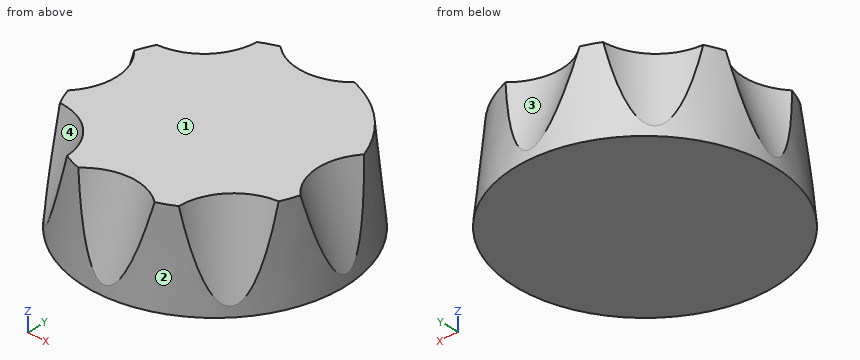
from build123d import *

# Parameters (mm, degrees)
REVOLVE1_ANGLE     = 19.5
CUT_EXTRUDE3_DEPTH = 30
REVOLVE2_ANGLE     = 19.5
CUT_EXTRUDE4_DEPTH = 30
REVOLVE3_ANGLE     = 19.5
CUT_EXTRUDE5_DEPTH = 30
REVOLVE4_ANGLE     = 19.5
CUT_EXTRUDE6_DEPTH = 30
REVOLVE5_ANGLE     = 19.5
CUT_EXTRUDE7_DEPTH = 30
REVOLVE6_ANGLE     = 19.5
CUT_EXTRUDE8_DEPTH = 30
REVOLVE7_ANGLE     = 19.5
CUT_EXTRUDE9_DEPTH = 30


# Read off the part's stored shape, not the designer's step: Boundary1
with BuildPart() as part:
    # Boundary1 outline → Boundary1 (revolve)
    with BuildSketch(Plane.XZ):
        Polygon((23.4, 0), (21.75, 16.55), (0, 16.55), (0, 0), align=None)
    revolve(axis=Axis((0, 0, 0), (0, 0, 1)))

    # Sketch3 → Revolve1 (revolve)
    with BuildSketch(Plane.XY.offset(16.55)):
        with BuildLine():
            ThreePointArc((6.7, 20.692329497), (0, 21.75), (-6.7, 20.692329497))
            ThreePointArc((-6.7, 20.692329497), (0, 18.897069907), (6.7, 20.692329497))
        make_face()
    revolve(axis=Axis((-21.75, 0, 16.55), (1, 0, 0)), revolution_arc=REVOLVE1_ANGLE)

    # Sketch21 → Cut-Extrude3 (cut)
    # profile 1 of 2: a face of its own
    with BuildSketch(Plane(origin=(0, -5.207626236, 14.705882831), x_dir=(1, 0, 0), z_dir=(0, -0.3338068592337716, 0.9426414910921781))):
        with BuildLine():
            Line((9.372530559, 28.241040631), (-9.372530559, 28.241040631))
            ThreePointArc((-9.372530559, 28.241040631), (0, 22.47450352), (9.372530559, 28.241040631))
        make_face()
        with BuildLine():
            ThreePointArc((6.7, 26.216833017), (0, 24.421573428), (-6.7, 26.216833017))
            ThreePointArc((-6.7, 26.216833017), (0, 27.27450352), (6.7, 26.216833017))
        make_face(mode=Mode.SUBTRACT)
    # profile 2 of 2: a face of its own
    with BuildSketch(Plane(origin=(0, -5.207626236, 14.705882831), x_dir=(1, 0, 0), z_dir=(0, -0.3338068592337716, 0.9426414910921781))):
        with BuildLine():
            ThreePointArc((6.7, 26.216833017), (0, 27.27450352), (-6.7, 26.216833017))
            ThreePointArc((-6.7, 26.216833017), (0, 24.421573428), (6.7, 26.216833017))
        make_face()
    extrude(amount=-CUT_EXTRUDE3_DEPTH, mode=Mode.SUBTRACT)

    # Sketch22 → Revolve2 (revolve)
    with BuildSketch(Plane.XY.offset(16.55)):
        with BuildLine():
            ThreePointArc((-19.454905378, 9.724667435), (-15.513197269, 15.244776499), (-10.062721237, 19.282223454))
            ThreePointArc((-10.062721237, 19.282223454), (-13.478343599, 13.245131366), (-19.454905378, 9.724667435))
        make_face()
    revolve(axis=Axis((-15.244776499, -15.513197269, 16.55), (0.7009092642998491, 0.7132504491541835, 0)), revolution_arc=REVOLVE2_ANGLE)

    # Sketch24 → Cut-Extrude4 (cut)
    with BuildSketch(Plane(origin=(3.714341752, -3.650073474, 14.705882831), x_dir=(0.971243492060928, 0.05687022863046558, -0.23119657485527895), z_dir=(0.23808789227923496, -0.23396832012378627, 0.9426414910921782))):
        with BuildLine():
            Line((-27.491870021, 14.371370891), (-13.585471932, 28.745378411))
            ThreePointArc((-13.585471932, 28.745378411), (-15.293280927, 16.483625521), (-27.491870021, 14.371370891))
        make_face()
    extrude(amount=-CUT_EXTRUDE4_DEPTH, mode=Mode.SUBTRACT)

    # Sketch25 → Revolve3 (revolve)
    with BuildSketch(Plane.XY.offset(16.55)):
        with BuildLine():
            ThreePointArc((-20.571898581, -7.061125177), (-21.74668737, -0.37958984), (-20.805796451, 6.338874823))
            ThreePointArc((-20.805796451, 6.338874823), (-18.893272141, -0.329783292), (-20.571898581, -7.061125177))
        make_face()
    revolve(axis=Axis((0.37958984, -21.74668737, 16.55), (-0.017452406437287054, 0.9998476951563913, 0)), revolution_arc=REVOLVE3_ANGLE)

    # Sketch26 → Cut-Extrude5 (cut)
    with BuildSketch(Plane(origin=(5.206833089, 0.09088561, 14.705882831), x_dir=(0.9426574907513692, -0.004123731024087582, -0.3337361981757048), z_dir=(0.33375601883228045, 0.00582573297890205, 0.9426414910921782))):
        with BuildLine():
            Line((-29.354887322, 9.164887842), (-30.256162535, -10.835112158))
            ThreePointArc((-30.256162535, -10.835112158), (-22.482645188, -1.165108658), (-29.354887322, 9.164887842))
        make_face()
    extrude(amount=-CUT_EXTRUDE5_DEPTH, mode=Mode.SUBTRACT)

    # Sketch27 → Revolve4 (revolve)
    with BuildSketch(Plane.XY.offset(16.55)):
        with BuildLine():
            ThreePointArc((-19.103667977, -10.397709836), (-14.971712021, -15.77689257), (-9.383651405, -19.621661151))
            ThreePointArc((-9.383651405, -19.621661151), (-13.007884538, -13.707450198), (-19.103667977, -10.397709836))
        make_face()
    revolve(axis=Axis((15.77689257, -14.971712021, 16.55), (-0.7253743710122916, 0.6883545756937498, 0)), revolution_arc=REVOLVE4_ANGLE)

    # Sketch28 → Cut-Extrude6 (cut)
    with BuildSketch(Plane(origin=(3.584693348, 3.777478605, 14.705882831), x_dir=(0.9732423250057362, -0.05845929079288866, -0.22222035941250265), z_dir=(0.2297774789515262, 0.24213494055628595, 0.9426414910921781))):
        with BuildLine():
            Line((-26.325903264, -15.059910067), (-12.852307992, -29.840377936))
            ThreePointArc((-12.852307992, -29.840377936), (-14.195389298, -17.533334095), (-26.325903264, -15.059910067))
        make_face()
    extrude(amount=-CUT_EXTRUDE6_DEPTH, mode=Mode.SUBTRACT)

    # Sketch29 → Revolve5 (revolve)
    with BuildSketch(Plane.XY.offset(16.55)):
        with BuildLine():
            ThreePointArc((-5.973766656, -20.913550917), (0.759064053, -21.736750488), (7.418070426, -20.445897661))
            ThreePointArc((7.418070426, -20.445897661), (0.659498229, -18.885558323), (-5.973766656, -20.913550917))
        make_face()
    revolve(axis=Axis((21.736750488, 0.759064053, 16.55), (-0.9993908270190959, -0.03489949670249739, 0)), revolution_arc=REVOLVE5_ANGLE)

    # Sketch30 → Cut-Extrude7 (cut)
    with BuildSketch(Plane(origin=(-0.181743535, 5.204453891, 14.705882831), x_dir=(0.9999321399924122, 0.0038771729275817748, 0.01098557874146117), z_dir=(-0.011649691383100024, 0.33360351311428743, 0.9426414910921777))):
        with BuildLine():
            Line((-9.086281711, -30.342992304), (10.880145152, -29.184632107))
            ThreePointArc((10.880145152, -29.184632107), (0.474220724, -22.477625897), (-9.086281711, -30.342992304))
        make_face()
    extrude(amount=-CUT_EXTRUDE7_DEPTH, mode=Mode.SUBTRACT)

    # Sketch31 → Revolve6 (revolve)
    with BuildSketch(Plane.XY.offset(16.55)):
        with BuildLine():
            ThreePointArc((19.782439975, -9.039777024), (16.035782076, -14.694087016), (10.729531193, -18.919293337))
            ThreePointArc((10.729531193, -18.919293337), (13.932381375, -12.766675382), (19.782439975, -9.039777024))
        make_face()
    revolve(axis=Axis((14.694087016, 16.035782076, 16.55), (-0.675590207615664, -0.7372773368101205, 0)), revolution_arc=REVOLVE6_ANGLE)

    # Sketch32 → Cut-Extrude8 (cut)
    with BuildSketch(Plane(origin=(-3.839464802, 3.51822129, 14.705882831), x_dir=(0.9692386501510535, 0.054574384261441185, 0.23999599087453166), z_dir=(-0.2461082321848259, 0.22551664533327645, 0.9426414910921782))):
        with BuildLine():
            Line((15.221586992, -29.008248881), (27.126990078, -12.937736215))
            ThreePointArc((27.126990078, -12.937736215), (15.309806614, -16.628450305), (15.221586992, -29.008248881))
        make_face()
    extrude(amount=-CUT_EXTRUDE8_DEPTH, mode=Mode.SUBTRACT)

    # Sketch33 → Revolve7 (revolve)
    with BuildSketch(Plane.XY.offset(16.55)):
        with BuildLine():
            ThreePointArc((20.313320471, 7.773770734), (21.720192381, 1.138307048), (21.014622285, -5.607865032))
            ThreePointArc((21.014622285, -5.607865032), (18.87117213, 0.988996224), (20.313320471, 7.773770734))
        make_face()
    revolve(axis=Axis((-1.138307048, 21.720192381, 16.55), (0.052335956242940865, -0.998629534754574, 0)), revolution_arc=REVOLVE7_ANGLE)

    # Sketch34 → Cut-Extrude9 (cut)
    with BuildSketch(Plane(origin=(-5.200489365, -0.272546099, 14.705882831), x_dir=(0.9427855723268154, -0.012319387513152558, 0.3331720235909673), z_dir=(-0.33334938853450696, -0.01747010117845218, 0.9426414910921781))):
        with BuildLine():
            Line((28.876049562, 11.693707416), (30.572326937, -8.234228831))
            ThreePointArc((30.572326937, -8.234228831), (22.452048009, 1.11073054), (28.876049562, 11.693707416))
        make_face()
    extrude(amount=-CUT_EXTRUDE9_DEPTH, mode=Mode.SUBTRACT)


solid = part.part
The model under review builds one solid part; all positions refer to its coordinate system, in mm. Face numbers are marked on the shaded views. Give positions to 0.01 mm unless a question says otherwise; leave off trailing zeros. Write item = value, one per line. Start each with the question number.
(1) For pin 1 Ø6 at (y, z) = (9, 2.5) entering from +X; pin 2 Ø1 at (y, z) = (2, 8.5) entering from -X; pin 3 Ø8 at (x, z) = (6, 9) entering from +Y, all flat-tipped, find the tip position at first contact; note any pin that passes through.
(2) Draft analysis for pull direction X (two halves, no side actions). For the marked faces 1, 2, 3 and 4, state which applies: +X half, -X half, draft (parallel to the pull), parting line (faces both ways), or undercut.
(3) For L1, parallel to X at y = 11.5, z = 4; L2, parallel to X at y = -13.5, z = 9.5; L3, parallel to Y at x = 15.5, z = 10.25, list the stretches that pass through material, from the lowest coordinate up. Write a range as from..to.
Returned:
q1.pin_1 = 22.42
q1.pin_2 = -21.39
q1.pin_3 = 22.53
q2.face_1 = draft
q2.face_2 = parting line
q2.face_3 = undercut
q2.face_4 = -X half
q3.L1 = -19.92..19.92
q3.L2 = -15.9..15.42
q3.L3 = -13.05..16.14
